Part model, mm, in its own coordinate system. A direction names the side the tool comes from. Coordinates: 2 decimals unless noted, no trailing zeros. Order: outer loops, then holes, each group sorted by start corner. A loop starts at its lowest first (then second) coordinate and runs counter-clockwise, first axis right, second up.
from build123d import *

# Parameters (mm, degrees)
SKETCH1_W                    = 6.35
SKETCH1_H                    = 2
BOSS_EXTRUDE1_DEPTH          = 12
SKETCH3_R                    = 10
BOSS_EXTRUDE2_DEPTH          = 9
F_5_0_5_DIAMETER_HOLE1_D     = 5
F_5_0_5_DIAMETER_HOLE1_DEPTH = 23


with BuildPart() as part:
    # Sketch1 → Revolve1 (revolve)
    with BuildSketch(Plane(origin=(0, 0, 0), x_dir=(1, 0, 0), z_dir=(0, 1, 0))):
        with Locations((3.175, -13)):
            Rectangle(SKETCH1_W, SKETCH1_H)
    revolve(axis=Axis((0, 0, 12), (0, 0, 1)))

    # Sketch2 → Boss-Extrude1 (add)
    with BuildSketch(Plane(origin=(0, 0, 12), x_dir=(-1, 0, 0), z_dir=(0, 0, -1))):
        with BuildLine():
            Line((-2.875186934, -4.932808292), (-2.337585335, -3.444483277))
            ThreePointArc((-2.337585335, -3.444483277), (-2.320135009, -3.243617805), (-2.400419134, -3.058669404))
            Line((-2.400419134, -3.058669404), (-3.024832437, -2.4306198))
            ThreePointArc((-3.024832437, -2.4306198), (-3.188663853, -2.33311555), (-3.378852537, -2.3198462))
            Line((-3.378852537, -2.3198462), (-4.867663341, -2.855580601))
            ThreePointArc((-4.867663341, -2.855580601), (-5.169157529, -2.882959187), (-5.446384241, -2.761329901))
            Line((-5.446384241, -2.761329901), (-5.807587241, -1.966542116))
            ThreePointArc((-5.807587241, -1.966542116), (-5.731084845, -1.673369369), (-5.521086391, -1.454958001))
            Line((-5.521086391, -1.454958001), (-4.088539945, -0.782695026))
            ThreePointArc((-4.088539945, -0.782695026), (-3.934167363, -0.653000933), (-3.860158544, -0.465453215))
            Line((-3.860158544, -0.465453215), (-3.857587291, 0.420171804))
            ThreePointArc((-3.857587291, 0.420171804), (-3.904487679, 0.604964025), (-4.029588541, 0.748830581))
            Line((-4.029588541, 0.748830581), (-5.461158184, 1.422757368))
            ThreePointArc((-5.461158184, 1.422757368), (-5.693706352, 1.61658637), (-5.803730347, 1.89862015))
            Line((-5.803730347, 1.89862015), (-5.497139595, 2.716029083))
            ThreePointArc((-5.497139595, 2.716029083), (-5.235739777, 2.86923814), (-4.93280828, 2.875186941))
            Line((-4.93280828, 2.875186941), (-3.444483265, 2.337585342))
            ThreePointArc((-3.444483265, 2.337585342), (-3.243617793, 2.320135016), (-3.058669391, 2.40041914))
            Line((-3.058669391, 2.40041914), (-2.430619781, 3.024832451))
            ThreePointArc((-2.430619781, 3.024832451), (-2.333115531, 3.188663866), (-2.319846181, 3.378852551))
            Line((-2.319846181, 3.378852551), (-2.855580582, 4.867663354))
            ThreePointArc((-2.855580582, 4.867663354), (-2.882959167, 5.169157543), (-2.761329882, 5.446384254))
            Line((-2.761329882, 5.446384254), (-1.966542082, 5.807587254))
            ThreePointArc((-1.966542082, 5.807587254), (-1.673369335, 5.731084833), (-1.454957982, 5.521086354))
            Line((-1.454957982, 5.521086354), (-0.782695007, 4.088539908))
            ThreePointArc((-0.782695007, 4.088539908), (-0.653000914, 3.934167326), (-0.465453196, 3.860158506))
            Line((-0.465453196, 3.860158506), (0.420171836, 3.857587254))
            ThreePointArc((0.420171836, 3.857587254), (0.604964057, 3.904487642), (0.748830613, 4.029588503))
            Line((0.748830613, 4.029588503), (1.4227574, 5.461158146))
            ThreePointArc((1.4227574, 5.461158146), (1.616586402, 5.693706315), (1.898620182, 5.80373031))
            Line((1.898620182, 5.80373031), (2.716029116, 5.497139558))
            ThreePointArc((2.716029116, 5.497139558), (2.869238173, 5.235739739), (2.875186973, 4.932808242))
            Line((2.875186973, 4.932808242), (2.337585375, 3.444483227))
            ThreePointArc((2.337585375, 3.444483227), (2.320135048, 3.243617755), (2.400419173, 3.058669354))
            Line((2.400419173, 3.058669354), (3.024832497, 2.43061973))
            ThreePointArc((3.024832497, 2.43061973), (3.188663912, 2.33311548), (3.378852597, 2.31984613))
            Line((3.378852597, 2.31984613), (4.8676634, 2.855580531))
            ThreePointArc((4.8676634, 2.855580531), (5.169157589, 2.882959117), (5.4463843, 2.761329831))
            Line((5.4463843, 2.761329831), (5.8075873, 1.966542031))
            ThreePointArc((5.8075873, 1.966542031), (5.731084879, 1.673369284), (5.5210864, 1.454957931))
            Line((5.5210864, 1.454957931), (4.088539954, 0.782694956))
            ThreePointArc((4.088539954, 0.782694956), (3.934167372, 0.653000863), (3.860158552, 0.465453145))
            Line((3.860158552, 0.465453145), (3.8575873, -0.420171864))
            ThreePointArc((3.8575873, -0.420171864), (3.904487688, -0.604964085), (4.029588549, -0.748830641))
            Line((4.029588549, -0.748830641), (5.461158192, -1.422757428))
            ThreePointArc((5.461158192, -1.422757428), (5.693706361, -1.616586429), (5.803730356, -1.898620209))
            Line((5.803730356, -1.898620209), (5.497139604, -2.716029143))
            ThreePointArc((5.497139604, -2.716029143), (5.235739785, -2.8692382), (4.932808288, -2.875187))
            Line((4.932808288, -2.875187), (3.444483273, -2.337585402))
            ThreePointArc((3.444483273, -2.337585402), (3.243617801, -2.320135075), (3.0586694, -2.4004192))
            Line((3.0586694, -2.4004192), (2.4306198, -3.0248325))
            ThreePointArc((2.4306198, -3.0248325), (2.33311555, -3.188663916), (2.3198462, -3.3788526))
            Line((2.3198462, -3.3788526), (2.855580601, -4.867663404))
            ThreePointArc((2.855580601, -4.867663404), (2.882959186, -5.169157592), (2.761329901, -5.446384304))
            Line((2.761329901, -5.446384304), (1.966542101, -5.807587304))
            ThreePointArc((1.966542101, -5.807587304), (1.673369354, -5.731084882), (1.454958001, -5.521086404))
            Line((1.454958001, -5.521086404), (0.782695026, -4.088539957))
            ThreePointArc((0.782695026, -4.088539957), (0.653000933, -3.934167376), (0.465453215, -3.860158556))
            Line((0.465453215, -3.860158556), (-0.420171797, -3.857587303))
            ThreePointArc((-0.420171797, -3.857587303), (-0.604964018, -3.904487692), (-0.748830574, -4.029588553))
            Line((-0.748830574, -4.029588553), (-1.422757361, -5.461158196))
            ThreePointArc((-1.422757361, -5.461158196), (-1.616586363, -5.693706365), (-1.898620143, -5.80373036))
            Line((-1.898620143, -5.80373036), (-2.716029077, -5.497139607))
            ThreePointArc((-2.716029077, -5.497139607), (-2.869238134, -5.235739789), (-2.875186934, -4.932808292))
        make_face()
    extrude(amount=BOSS_EXTRUDE1_DEPTH)

    # Sketch3 → Boss-Extrude2 (add)
    with BuildSketch(Plane.XY):
        Circle(SKETCH3_R)
    extrude(amount=-BOSS_EXTRUDE2_DEPTH)

    # Ø5.0 (5) Diameter Hole1
    with Locations(Plane(origin=(0, 0, -9), x_dir=(-1, 0, 0), z_dir=(0, 0, -1))):
        with Locations((0, 0)):
            Hole(F_5_0_5_DIAMETER_HOLE1_D / 2, depth=F_5_0_5_DIAMETER_HOLE1_DEPTH)


solid = part.part
Q1. Pin check, flat tips, straight feed: pin 1 Ø6 at (y, z) = (-2, 10.5) entering from -X; pin 2 Ø1.5 at (y, z) = (-5, 2.5) entering from -X; pin 3 Ø3 at (x, z) = (3, 5.5) entering from -Y; pin 4 Ø3 at (x, z) = (7.5, 10.5) entering from -Y. Stop position of each tip, or through.
Results list:
pin 1: stops at x = -6.35
pin 2: stops at x = -2.89
pin 3: stops at y = -5.8
pin 4: passes through
Q2. Wall check: line 1 along Z through (x, y) = (-0.5, 4.5); line 2 along Y through (x, z) = (0, -1.5); line 3 along Y through (x, z) = (0, 5.5). Give the ranges that are in metal, low to high.
Results list:
line 1: z = -9 to 0, 12 to 14
line 2: y = -10 to -2.5, 2.5 to 10
line 3: y = -3.86 to -2.5, 2.5 to 3.86
Q3. Which spindle directions (+Z, -Z, +X, -X, +Y, -Y) get a long thin tool onto all of the face, cutting with end or side? Do faces 1 (the face through (-2.302, 5.653, 6.084)), 2 (the face through (-4.2, -2.61, 6.08)), 3 (the face through (-3, -3, 12)), 4 (the face through (4.735, 1.081, 6.084)). Say none if no direction does.
Results list:
face 1: -X, +Y
face 2: -Y
face 3: none
face 4: +X
Q4. Cut at A-A on x = 0. Write the cut outline in (y, z), and give its area (3 significant figures).
Results list:
outline: (-10, -9) - (-2.5, -9) - (-2.5, 14) - (-6.35, 14) - (-6.35, 12) - (-3.86, 12) - (-3.86, 0) - (-10, 0) - close; (2.5, -9) - (10, -9) - (10, 0) - (3.86, 0) - (3.86, 12) - (6.35, 12) - (6.35, 14) - (2.5, 14) - close
area: 183 mm2
Q5. Cut at C-C on z = -6.25. Write the cut outline in (x, y).
Results list:
outline: circle Ø20 at (0, 0); hole circle Ø5 at (0, 0)
Q6. Cut at D-D on y = -8.25. Write the cut outline in (x, z).
Results list:
outline: (-5.65, -9) - (5.65, -9) - (5.65, 0) - (-5.65, 0) - close
Q7. Mould opens along Z. For faces 5 (the face through (-0.54, -2.44, 2.66)), 6 (the face through (4.113, -2.584, 6.084)), 7 (the face through (2, -2, -9)) say: pulls with the +Z half, pulls with the -Z half, needs draft (parallel to the pull), parting line crosses it, or undercut.
Results list:
face 5: needs draft
face 6: undercut
face 7: pulls with the -Z half
